from build123d import *

# Parameters (mm, degrees)
SKETCH054_R           = 36.5
PAD024_DEPTH          = 37
SKETCH055_W           = 42
SKETCH055_H           = 42
POCKET015_DEPTH       = 7
SKETCH056_R           = 32.5
POCKET016_DEPTH       = 27
SKETCH057_R           = 15
POCKET017_DEPTH       = 5
SKETCH058_R           = 1.5
POCKET018_DEPTH       = 5
POLARPATTERN004_COUNT = 4
PAD025_DEPTH          = 37
SKETCH060_W           = 42
SKETCH060_H           = 21
POCKET019_DEPTH       = 30
SKETCH061_W           = 18
SKETCH061_H           = 15
POCKET020_DEPTH       = 5
SKETCH062_W           = 25
SKETCH062_H           = 42
POCKET021_DEPTH       = 10
SKETCH064_R           = 2.5
POCKET023_DEPTH       = 81.501
SKETCH065_R           = 2.5
POCKET024_DEPTH       = 37.001


with BuildPart() as part:
    # Sketch054 → Pad024 (new body)
    with BuildSketch(Plane.XY):
        Circle(SKETCH054_R)
    extrude(amount=PAD024_DEPTH)

    # Sketch055 (on Face3 of Pad024) → Pocket015 (cut)
    with BuildSketch(Plane.XY.offset(37)):
        Rectangle(SKETCH055_W, SKETCH055_H)
    extrude(amount=-POCKET015_DEPTH, mode=Mode.SUBTRACT)

    # Sketch056 (on Face2 of Pocket015) → Pocket016 (cut)
    with BuildSketch(Plane(origin=(0, 0, 0), x_dir=(1, 0, 0), z_dir=(0, 0, -1))):
        Circle(SKETCH056_R)
    extrude(amount=-POCKET016_DEPTH, mode=Mode.SUBTRACT)

    # Sketch057 (on Face9 of Pocket016) → Pocket017 (cut)
    with BuildSketch(Plane(origin=(0, 0, 27), x_dir=(1, 0, 0), z_dir=(0, 0, -1))):
        Circle(SKETCH057_R)
    extrude(amount=-POCKET017_DEPTH, mode=Mode.SUBTRACT)

    # Sketch058 (on Face9 of Pocket017) → Pocket018 (cut)
    with BuildSketch(Plane(origin=(0, 0, 27), x_dir=(1, 0, 0), z_dir=(0, 0, -1))):
        with Locations((-15.5, 15.5)):
            Circle(SKETCH058_R)
    pocket018 = extrude(amount=-POCKET018_DEPTH, mode=Mode.SUBTRACT)

    # PolarPattern004: Pocket018 ×4 about axis
    polarpattern004_axis = Axis((0, 0, 27), (0, 0, -1))
    for i in range(1, POLARPATTERN004_COUNT):
        add(pocket018.rotate(polarpattern004_axis, i * 360 / POLARPATTERN004_COUNT), mode=Mode.SUBTRACT)

    # Sketch059 (on Face2 of PolarPattern004) → Pad025 (join)
    with BuildSketch(Plane(origin=(0, 0, 0), x_dir=(1, 0, 0), z_dir=(0, 0, -1))):
        with BuildLine():
            Line((-45, 27), (-45, -27))
            Line((-45, -27), (-24.561148, -27))
            ThreePointArc((-24.561148, 27), (-36.5, 0), (-24.561148, -27))
            Line((-45, 27), (-24.561148, 27))
        make_face()
    extrude(amount=-PAD025_DEPTH)

    # Sketch060 (on Face2 of Pad025) → Pocket019 (cut)
    with BuildSketch(Plane(origin=(-40, 0, 0), x_dir=(0, -1, 0), z_dir=(-1, 0, 0))):
        with Locations((0, 16.5)):
            Rectangle(SKETCH060_W, SKETCH060_H)
    extrude(amount=-POCKET019_DEPTH, mode=Mode.SUBTRACT)

    # Sketch061 (on Face2 of Pocket019) → Pocket020 (cut)
    with BuildSketch(Plane(origin=(-45, 0, 0), x_dir=(0, -1, 0), z_dir=(-1, 0, 0))):
        with Locations((0, 16.5)):
            Rectangle(SKETCH061_W, SKETCH061_H)
    extrude(amount=-POCKET020_DEPTH, mode=Mode.SUBTRACT)

    # Sketch062 (on Face4 of Pocket020) → Pocket021 (cut)
    with BuildSketch(Plane(origin=(0, 0, 0), x_dir=(1, 0, 0), z_dir=(0, 0, -1))):
        with Locations((-27.5, 0)):
            Rectangle(SKETCH062_W, SKETCH062_H)
    extrude(amount=-POCKET021_DEPTH, mode=Mode.SUBTRACT)

    # Sketch064 (on Face2 of Pocket021) → Pocket023 (cut, through all)
    with BuildSketch(Plane(origin=(-45, 0, 0), x_dir=(0, -1, 0), z_dir=(-1, 0, 0))):
        with Locations((-14, 22)):
            Circle(SKETCH064_R)
        with Locations((14, 22)):
            Circle(SKETCH064_R)
        with Locations((14, 7.436279)):
            Circle(SKETCH064_R)
        with Locations((-14, 7.436279)):
            Circle(SKETCH064_R)
    extrude(amount=-POCKET023_DEPTH, mode=Mode.SUBTRACT)

    # Sketch065 (on Face5 of Pocket023) → Pocket024 (cut, through all)
    with BuildSketch(Plane.XY.offset(37)):
        with Locations((27, 0)):
            Circle(SKETCH065_R)
        with Locations((0, 27)):
            Circle(SKETCH065_R)
        with Locations((0, -27)):
            Circle(SKETCH065_R)
        with Locations((-27, 0)):
            Circle(SKETCH065_R)
    extrude(amount=-POCKET024_DEPTH, mode=Mode.SUBTRACT)


with BuildPart() as part_1:
    # Body005 placement: moved
    add(part.part.moved(Location((260.222748, 1.6e-05, -14.462208))))


solid = part_1.part
Check sheet for the modelled part. Datum: model origin and axes. Units: mm. A direction names the side the tool comes from. Round coordinates to 2 decimals unless told otherwise and drop trailing zeros. Write each loop counter-clockwise with the first axis right and the second up, starting at its lowest first coordinate (ties: lowest second). Pieces come first, ordered by that corner, then holes. Notation, with made-up numbers: (27, -11) - (86, -11) arc R30 cw to (86, 26) - close; hole circle Ø2 at (80, 75.25). An arc over 180 degrees is marked (long way). Return JSON: item names as keys, results as strings.
Q1. Cross-section at A-A (x = 251). Record the boundary of the cut face in (y, z), then the cut area to 3 significant figures.
Returned:
{"outline": "(-35.32, -14.46) - (-31.16, -14.46) - (-31.16, 12.54) - (-11.83, 12.54) - (-11.83, 15.54) - (-21, 15.54) - (-21, 22.54) - (-35.32, 22.54) - close; (11.83, 12.54) - (31.16, 12.54) - (31.16, -14.46) - (35.32, -14.46) - (35.32, 22.54) - (21, 22.54) - (21, 15.54) - (11.83, 15.54) - close", "area": "566 mm²"}
Q2. Cross-section at B-B (y = -8). Record the boundary of the cut face in (x, z).
Returned:
{"outline": "(215.22, -14.46) - (220.22, -14.46) - (220.22, -5.46) - (215.22, -5.46) - close; (215.22, 9.54) - (220.22, 9.54) - (220.22, 12.54) - (247.53, 12.54) - (247.53, 15.54) - (239.22, 15.54) - (239.22, 22.54) - (215.22, 22.54) - close; (272.91, 12.54) - (291.72, 12.54) - (291.72, -14.46) - (295.84, -14.46) - (295.84, 22.54) - (281.22, 22.54) - (281.22, 15.54) - (272.91, 15.54) - close"}
Q3. Cross-section at C-C (y = 25.5). Record the boundary of the cut face in (x, z), then the cut area to 3 significant figures.
Returned:
{"outline": "(215.22, -14.46) - (240.07, -14.46) - (240.07, 12.54) - (258.22, 12.54) - (258.22, 22.54) - (215.22, 22.54) - close; (262.22, 12.54) - (280.37, 12.54) - (280.37, -14.46) - (286.34, -14.46) - (286.34, 22.54) - (262.22, 22.54) - close", "area": "1,500 mm²"}
Q4. Access from +Z, -Z, +X, -X, +Y, -Y to the whole of each face (thin tool, end or side, straight path). Record for faces 4 (the flat face through (228, -21, -1)), 5 (the flat face through (218, 9, 2)), 6 (the flat face through (260, 21, 19)).
Returned:
{"face 4": "-Z", "face 5": "-X", "face 6": "+Z"}
Q5. Cross-section at D-D (x = 241.5). Record the boundary of the cut face in (y, z).
Returned:
{"outline": "(-31.33, -14.46) - (-26.57, -14.46) - (-26.57, 12.54) - (26.57, 12.54) - (26.57, -14.46) - (31.33, -14.46) - (31.33, 22.54) - (21, 22.54) - (21, 15.54) - (-21, 15.54) - (-21, 22.54) - (-31.33, 22.54) - close"}
Q6. Draft check along Z on faces 1 (the flat face through (218, -9, 2)), 2 (the flat face through (245.9, 5, 15.538)), 3 (the cylindrical face through (245.237, -0.66, 14.017)). Enter one of: released by +Z, released by -Z, zero draft, split by the parting line, or undercut.
Returned:
{"face 1": "undercut", "face 2": "released by +Z", "face 3": "zero draft"}
Q7. Depth check by flat-ended pin: P1, Ø5, axis at x = 271, y = 11, coming from the +Z side; P2, Ø4.5, axis at y = -14, z = 7.54, coming from the +X side; P3, Ø10, axis at x = 276, y = -21, coming from the -Z side; P4, Ø2, axis at x = 266, z = 19.5, coming from the +Y side. Enter the tip coordinate at first touch or a pass-through.
Returned:
{"P1": "stops at z = 15.54", "P2": "passes through", "P3": "stops at z = 12.54", "P4": "stops at y = 36.19"}
Q8. Scan lines: L1, parallel to Y at x = 220.5, z = 5.5; L2, parallel to Y at x = 260, z = -12.5; L3, parallel to Y at x = 230, z = 13. Record each from-to range of solid material in increasing order. Write a range as from..to.
Returned:
{"L1": "y = -27..-21, 21..27", "L2": "y = -36.5..-32.5, 32.5..36.5", "L3": "y = -27..27"}
